Build history of the part. All positions in model axes, mm. Face numbers are marked on the shaded views. A direction names the side the tool comes from. Coordinates: 2 decimals unless noted, no trailing zeros. Order: outer loops, then holes, each group sorted by start corner. A loop starts at its lowest first (then second) coordinate and runs counter-clockwise, first axis right, second up. Notation, with made-up numbers: (-22.75, 64.5) - (-15.75, 64.5) arc R35 ccw to (-15.75, 98.5) - close; hole circle Ø4 at (58, 40.5). An arc over 180 degrees is marked (long way). Return JSON: item names as keys, results as strings.
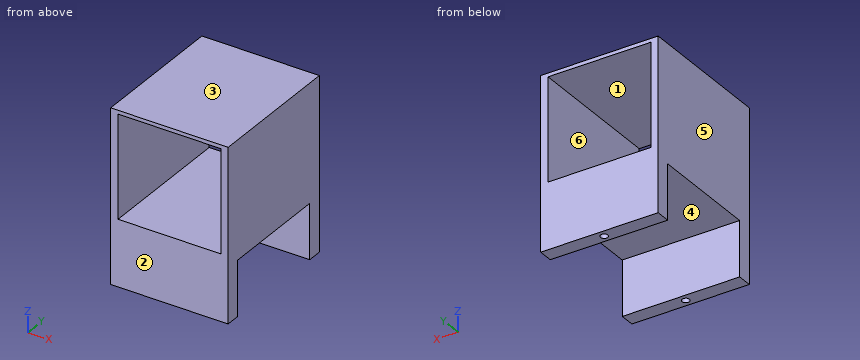
from build123d import *

# Parameters (mm, degrees)
BOSS_EXTRUDE1_DEPTH = 16
SKETCH2_W           = 28
SKETCH2_H           = 28
CUT_EXTRUDE1_DEPTH  = 39
SKETCH3_R           = 1
CUT_EXTRUDE2_DEPTH  = 2


with BuildPart() as part:
    # Sketch1 → Boss-Extrude1 (new body, symmetric)
    with BuildSketch(Plane(origin=(0, 0, 0), x_dir=(0, 0, -1), z_dir=(1, 0, 0))):
        Polygon((0, 0), (0, 38), (47, 38), (47, 34), (32, 34), (32, 4), (47, 4), (47, 0), align=None)
    extrude(amount=BOSS_EXTRUDE1_DEPTH, both=True)

    # Sketch2 → Cut-Extrude1 (cut, through all)
    with BuildSketch(Plane(origin=(0, 38, 0), x_dir=(1, 0, 0), z_dir=(0, 1, 0))):
        with Locations((0, 15)):
            Rectangle(SKETCH2_W, SKETCH2_H)
    extrude(amount=-CUT_EXTRUDE1_DEPTH, mode=Mode.SUBTRACT)

    # Sketch3 → Cut-Extrude2 (cut)
    with BuildSketch(Plane(origin=(0, 0, -47), x_dir=(-1, 0, 0), z_dir=(0, 0, -1))):
        with Locations((0, 36)):
            Circle(SKETCH3_R)
        with Locations((0, 2)):
            Circle(SKETCH3_R)
    extrude(amount=-CUT_EXTRUDE2_DEPTH, mode=Mode.SUBTRACT)


solid = part.part
1. Probe L1, parallel to Y at x = 0, z = -45.45; L2, parallel to Z at x = 10.5, y = 14; L3, parallel to Z at x = -3, y = 35.5. List the from-to ranges inside material, lowest first.
Check values:
{"L1": "0 to 1, 3 to 4, 34 to 35, 37 to 38", "L2": "-32 to -29, -1 to 0", "L3": "-47 to -29, -1 to 0"}
2. Mould opens along Z. For the marked faces 1, 2 and 3 say: pulls with the +Z half, pulls with the -Z half, needs draft (parallel to the pull), parting line crosses it, or undercut.
Check values:
{"face 1": "undercut", "face 2": "needs draft", "face 3": "pulls with the +Z half"}
3. Cut at C-C on y = 10.5. Give the cut face in (x, z), plus the area to 3 significant figures.
Check values:
{"outline": "(-16, -32) - (16, -32) - (16, 0) - (-16, 0) - close; hole (-14, -29) - (14, -29) - (14, -1) - (-14, -1) - close", "area": "240 mm²"}
4. Cut at B-B on x = 0. Give the cut face in (y, z).
Check values:
{"outline": "(0, -47) - (1, -47) - (1, -45) - (3, -45) - (3, -47) - (4, -47) - (4, -32) - (34, -32) - (34, -47) - (35, -47) - (35, -45) - (37, -45) - (37, -47) - (38, -47) - (38, -29) - (0, -29) - close; (0, -1) - (38, -1) - (38, 0) - (0, 0) - close"}
5. Tool access for the marked faces 4, 5 and 6: list every direction of +Z, -Z, +X, -X, +Y, -Y with a clear straight run to the whole face (end or side of a thin tool).
Check values:
{"face 4": "-Z, +X, -X", "face 5": "+Z, -Z, -X, +Y, -Y", "face 6": "+Y, -Y"}
6. Cut at A-A on z = -21.5. Give the cut face in (x, y).
Check values:
{"outline": "(-16, 0) - (-14, 0) - (-14, 38) - (-16, 38) - close; (14, 0) - (16, 0) - (16, 38) - (14, 38) - close"}
7. Cut at D-D on x = 12. Give the cut face in (y, z), plus the area to 3 significant figures.
Check values:
{"outline": "(0, -47) - (4, -47) - (4, -32) - (34, -32) - (34, -47) - (38, -47) - (38, -29) - (0, -29) - close; (0, -1) - (38, -1) - (38, 0) - (0, 0) - close", "area": "272 mm²"}
8. Drop flat-ended pins along their axis: pin 1 (3 mm diameter, centred on x = 2.5, z = -40.5, fed in from -Y); pin 2 (8 mm diameter, centred on x = -7.5, z = -24, fed in from +Y); pin 3 (1.2 mm diameter, centred on x = 0, y = 36, fed in from -Z); pin 4 (15 mm diameter, centred on x = -6.5, y = 18.5, fed in from -Z). Give the stop position or say it passes through.
Check values:
{"pin 1": "y = 0", "pin 2": "through", "pin 3": "z = -45", "pin 4": "z = -32"}
